```python
from build123d import *

# Parameters (mm, degrees)
SKETCH1_W           = 33.909
SKETCH1_H           = 50.8
BOSS_EXTRUDE1_DEPTH = 76.2
CUT_EXTRUDE1_REACH  = 89.186
SKETCH2_R           = 6.731
SKETCH3_R           = 9.906
CUT_EXTRUDE2_DEPTH  = 28.956
SKETCH4_W           = 4.494494968
SKETCH4_H           = 6.35
CUT_EXTRUDE4_DEPTH  = 156.42964669
SKETCH5_W           = 152.4
SKETCH5_H           = 6.35
CUT_EXTRUDE5_DEPTH  = 12.7


with BuildPart() as part:
    # Sketch1 → Boss-Extrude1 (new, symmetric)
    with BuildSketch(Plane.XY):
        Rectangle(SKETCH1_W, SKETCH1_H)
    extrude(amount=BOSS_EXTRUDE1_DEPTH, both=True)

    # Sketch2 → Cut-Extrude1 (cut, up to next)
    with BuildSketch(Plane(origin=(16.9545, 0, 0), x_dir=(0, 0, -1), z_dir=(1, 0, 0)), mode=Mode.PRIVATE) as cut_extrude1_sk1:
        with Locations((-49.2125, -1.524)):
            Circle(SKETCH2_R)
    cut_extrude1_tool1 = extrude(cut_extrude1_sk1.sketch, amount=-CUT_EXTRUDE1_REACH, mode=Mode.PRIVATE) & part.part
    # Sketch2 → Cut-Extrude1 (cut, up to next)
    with BuildSketch(Plane(origin=(16.9545, 0, 0), x_dir=(0, 0, -1), z_dir=(1, 0, 0)), mode=Mode.PRIVATE) as cut_extrude1_sk2:
        with Locations((49.2125, -1.524)):
            Circle(SKETCH2_R)
    cut_extrude1_tool2 = extrude(cut_extrude1_sk2.sketch, amount=-CUT_EXTRUDE1_REACH, mode=Mode.PRIVATE) & part.part
    add(cut_extrude1_tool1.solids().sort_by_distance((16.9545, -1.524, 49.2125))[0], mode=Mode.SUBTRACT)
    add(cut_extrude1_tool2.solids().sort_by_distance((16.9545, -1.524, -49.2125))[0], mode=Mode.SUBTRACT)

    # Sketch3 → Cut-Extrude2 (cut)
    with BuildSketch(Plane(origin=(16.9545, 0, 0), x_dir=(0, 0, -1), z_dir=(1, 0, 0))):
        with Locations((-49.2125, -1.524)):
            Circle(SKETCH3_R)
        with Locations((49.2125, -1.524)):
            Circle(SKETCH3_R)
    extrude(amount=-CUT_EXTRUDE2_DEPTH, mode=Mode.SUBTRACT)

    # Sketch4 → Cut-Extrude4 (cut, through all)
    with BuildSketch(Plane.XY.offset(76.2)):
        with Locations((14.707252516, -22.225)):
            Rectangle(SKETCH4_W, SKETCH4_H)
    extrude(amount=-CUT_EXTRUDE4_DEPTH, mode=Mode.SUBTRACT)

    # Sketch5 → Cut-Extrude5 (cut)
    with BuildSketch(Plane(origin=(16.9545, 0, 0), x_dir=(0, 0, -1), z_dir=(1, 0, 0))):
        with Locations((0, -22.225)):
            Rectangle(SKETCH5_W, SKETCH5_H)
    extrude(amount=-CUT_EXTRUDE5_DEPTH, mode=Mode.SUBTRACT)


solid = part.part
```
For this review, take the finished solid that the model builds, in its own axes (mm). A direction names the side the tool comes from. Coordinates: 2 decimals unless noted, no trailing zeros. Write each loop counter-clockwise with the first axis right and the second up, starting at its lowest first coordinate (ties: lowest second). Pieces come first, ordered by that corner, then holes. Notation, with made-up numbers: (-3.75, 80) - (37.25, 80) arc R19 cw to (37.25, 91) - close; hole circle Ø4 at (2.25, -23). An arc over 180 degrees is marked (long way). Answer in a Markdown table with one row per item. Add a question column.
Q1. For probe 1 along Z at (x, y) = (-13.5, 0); probe 2 along Z at (x, y) = (6, 4.5); probe 3 along Y at (x, z) = (9.5, -67), list the stretches that pass through material, from the lowest coordinate up.
Q2. We need section A-A, the plane z = -13.5. State the section outline as (x, y) points, and give its area (3 significant figures).
Q3. We need section D-D, the plane x = 7. State the section outline as (y, z) points.
Q4. We need section C-C, the plane z = -49. State the section outline as (x, y) points.
Q5. Tool access review of faces 5 (the flat face through (11, -19.05, 1)), 6 (the flat face through (-12.002, -4, -56)), 7 (the flat face through (16.954, 3, 1)): name each direction out of +Z, -Z, +X, -X, +Y, -Y from which nothing blocks a thin tool from reaching the whole face with its end or side.
Q6. We need section B-B, the plane x = -8.5. State the section outline as (y, z) points, and give its area (3 significant figures).
Q7. For P1, Ø18, axis at y = -1.52, z = -49.21, coming from the +X side; P2, Ø5, axis at x = 10.5, z = -38.5, coming from the -Y side; P3, Ø7, axis at y = -23, z = 14, coming from the +X side, all flat-tipped, find the tip position at first contact; note any pin that passes through.
Q8. Draft analysis for pull direction Z (two halves, no side actions). For faces 1 (the flat face through (0, 0, 76.2)), 2 (the cylindrical face through (-14.443, -4.102, 42.995)), 3 (the cylindrical face through (-14.44, -4.1, -55.43)), 4 (the flat face through (0, 25.4, 1)), state which applies: +Z half, -Z half, draft (parallel to the pull), parting line (faces both ways), or undercut.
Answer list:
| question | item | result |
|---|---|---|
| 1 | probe 1 | z = -76.2 to -55.77, -42.66 to 42.66, 55.77 to 76.2 |
| 1 | probe 2 | z = -76.2 to -57.08, -41.35 to 41.35, 57.08 to 76.2 |
| 1 | probe 3 | y = -19.05 to 25.4 |
| 2 | outline | (-16.95, -25.4) - (4.25, -25.4) - (4.25, -19.05) - (16.95, -19.05) - (16.95, 25.4) - (-16.95, 25.4) - close |
| 2 | area | 1,640 mm2 |
| 3 | outline | (-19.05, -76.2) - (25.4, -76.2) - (25.4, 76.2) - (-19.05, 76.2) - close; hole circle Ø19.81 at (-1.52, -49.21); hole circle Ø19.81 at (-1.52, 49.21) |
| 4 | outline | (-16.95, -25.4) - (4.25, -25.4) - (4.25, -19.05) - (16.95, -19.05) - (16.95, -11.43) - (-12, -11.43) - (-12, -8.25) - (-16.95, -8.25) - close; (-16.95, 5.2) - (-12, 5.2) - (-12, 8.38) - (16.95, 8.38) - (16.95, 25.4) - (-16.95, 25.4) - close |
| 5 | face 5 | +Z, -Z, +X, -Y |
| 5 | face 6 | +X |
| 5 | face 7 | +Z, -Z, +X, +Y, -Y |
| 6 | outline | (-25.4, -76.2) - (25.4, -76.2) - (25.4, 76.2) - (-25.4, 76.2) - close; hole circle Ø19.81 at (-1.52, -49.21); hole circle Ø19.81 at (-1.52, 49.21) |
| 6 | area | 7,130 mm2 |
| 7 | P1 | stops at x = -12 |
| 7 | P2 | stops at y = -19.05 |
| 7 | P3 | stops at x = 4.25 |
| 8 | face 1 | +Z half |
| 8 | face 2 | undercut |
| 8 | face 3 | undercut |
| 8 | face 4 | draft |
